Build history of the part. All positions in model axes, mm. A direction names the side the tool comes from. Round coordinates to 2 decimals unless told otherwise and drop trailing zeros. Order: outer loops, then holes, each group sorted by start corner. A loop starts at its lowest first (then second) coordinate and runs counter-clockwise, first axis right, second up. Notation, with made-up numbers: (59, 46.5) -> (89, 46.5) arc R24 ccw to (89, 76.5) -> close; hole circle Ø8 at (58.5, 77.5). An arc over 180 degrees is marked (long way). Answer as a JSON object with one key per item and string values.
from build123d import *

# Parameters (mm, degrees)
SKETCH_W        = 60
SKETCH_H        = 30
PAD_DEPTH       = 18
SKETCH001_W     = 16
SKETCH001_H     = 22
POCKET_DEPTH    = 15
SKETCH002_W     = 16
SKETCH002_H     = 10
POCKET001_DEPTH = 5
SKETCH003_R     = 2.3
POCKET002_DEPTH = 10
FILLET_R        = 5
CHAMFER_SIZE    = 4
CHAMFER001_SIZE = 0.6
CHAMFER002_SIZE = 1
SKETCH004_R     = 4
POCKET003_DEPTH = 5
CHAMFER003_SIZE = 0.4
FILLET001_R     = 1


with BuildPart() as part:
    # Sketch (on XZ_Plane of Origin) → Pad (new body)
    with BuildSketch(Plane.XZ):
        Rectangle(SKETCH_W, SKETCH_H)
    extrude(amount=PAD_DEPTH)

    # Sketch001 (on Face6 of Pad) → Pocket (cut)
    with BuildSketch(Plane.XZ.offset(18)):
        with Locations((-10, -1)):
            Rectangle(SKETCH001_W, SKETCH001_H)
        with Locations((10, -1)):
            Rectangle(SKETCH001_W, SKETCH001_H)
    extrude(amount=-POCKET_DEPTH, mode=Mode.SUBTRACT)

    # Sketch002 (on Face13 of Pocket) → Pocket001 (cut)
    with BuildSketch(Plane.XY.offset(-12)):
        with Locations((-10, -13)):
            Rectangle(SKETCH002_W, SKETCH002_H)
        with Locations((10, -13)):
            Rectangle(SKETCH002_W, SKETCH002_H)
    extrude(amount=-POCKET001_DEPTH, mode=Mode.SUBTRACT)

    # Sketch003 (on Face4 of Pocket001) → Pocket002 (cut)
    with BuildSketch(Plane.XZ.offset(18)):
        with Locations((-24, 0)):
            Circle(SKETCH003_R)
        with Locations((24, 0)):
            Circle(SKETCH003_R)
    extrude(amount=-POCKET002_DEPTH, mode=Mode.SUBTRACT)

    # Fillet
    fillet_edges = [part.edges().sort_by_distance(p)[0] for p in [
        (30, -9, -15),
        (30, -9, 15),
        (-30, -9, 15),
        (-30, -9, -15),
    ]]
    fillet(fillet_edges, radius=FILLET_R)

    # Chamfer
    chamfer_edges = [part.edges().sort_by_distance(p)[0] for p in [
        (0, -18, -15),
    ]]
    chamfer(chamfer_edges, length=CHAMFER_SIZE)

    # Chamfer001
    chamfer001_edges = [part.edges().sort_by_distance(p)[0] for p in [
        (-26.3, -18, 0),
        (21.7, -18, 0),
    ]]
    chamfer(chamfer001_edges, length=CHAMFER001_SIZE)

    # Chamfer002
    chamfer002_edges = [part.edges().sort_by_distance(p)[0] for p in [
        (-21.5, -18, -15),
    ]]
    chamfer(chamfer002_edges, length=CHAMFER002_SIZE)

    # Sketch004 → Pocket003 (cut)
    with BuildSketch(Plane.XZ.offset(3)):
        with Locations((-10, 0)):
            Circle(SKETCH004_R)
        with Locations((10, 0)):
            Circle(SKETCH004_R)
    extrude(amount=-POCKET003_DEPTH, mode=Mode.SUBTRACT)

    # Chamfer003
    chamfer003_edges = [part.edges().sort_by_distance(p)[0] for p in [
        (0, 0, -15),
        (-28.535534, 0, -13.535534),
        (28.535534, 0, -13.535534),
        (-30, 0, 0),
        (30, 0, 0),
        (-28.535534, 0, 13.535534),
        (28.535534, 0, 13.535534),
        (0, 0, 15),
        (-14, 0, 0),
        (6, 0, 0),
    ]]
    chamfer(chamfer003_edges, length=CHAMFER003_SIZE)

    # Fillet001
    fillet001_edges = [part.edges().sort_by_distance(p)[0] for p in [
        (-2, -10.5, 10),
        (2, -10.5, 10),
        (18, -10.5, 10),
        (-18, -10.5, 10),
    ]]
    fillet(fillet001_edges, radius=FILLET001_R)


solid = part.part
1) Cut at D-D, the plane x = -24. Give the cut face in (y, z).
Checked values:
{"outline": "(-18, -14) -> (-17, -15) -> (-0.4, -15) -> (0, -14.6) -> (0, 14.6) -> (-0.4, 15) -> (-17, 15) -> (-18, 14) -> (-18, 2.9) -> (-17.4, 2.3) -> (-8, 2.3) -> (-8, -2.3) -> (-17.4, -2.3) -> (-18, -2.9) -> close"}
2) Cut at C-C, the plane y = -15. Give the cut face in (x, z).
Checked values:
{"outline": "(-30, -10) arc R5 ccw to (-25, -15) -> (-18, -15) -> (-18, 9) arc R1 cw to (-17, 10) -> (-3, 10) arc R1 cw to (-2, 9) -> (-2, -14) -> (2, -14) -> (2, 9) arc R1 cw to (3, 10) -> (17, 10) arc R1 cw to (18, 9) -> (18, -15) -> (25, -15) arc R5 ccw to (30, -10) -> (30, 10) arc R5 ccw to (25, 15) -> (-25, 15) arc R5 ccw to (-30, 10) -> close; hole circle Ø4.6 at (-24, 0); hole circle Ø4.6 at (24, 0)"}
3) Cut at A-A, the plane y = -4.5. Give the cut face in (x, z), plus the area to 3 significant figures.
Checked values:
{"outline": "(-30, -10) arc R5 ccw to (-25, -15) -> (25, -15) arc R5 ccw to (30, -10) -> (30, 10) arc R5 ccw to (25, 15) -> (-25, 15) arc R5 ccw to (-30, 10) -> close; hole (-18, -12) -> (-2, -12) -> (-2, 9) arc R1 ccw to (-3, 10) -> (-17, 10) arc R1 ccw to (-18, 9) -> close; hole (2, -12) -> (18, -12) -> (18, 9) arc R1 ccw to (17, 10) -> (3, 10) arc R1 ccw to (2, 9) -> close", "area": "1,080 mm²"}
4) Pull direction Z, two halves, no side cores. Call faces 1 (the face through (-27.996, -17.715, 13.063)), 2 (the face through (0, 0, 0)), 3 (the face through (6, -2, 0)): pulls with the +Z half, pulls with the -Z half, needs draft (parallel to the pull), parting line crosses it, or undercut.
Checked values:
{"face 1": "pulls with the +Z half", "face 2": "needs draft", "face 3": "undercut"}
5) Probe L1, parallel to X at y = -8.25, z = -5.75; L2, parallel to Z at x = 24, y = -14; L3, parallel to Z at x = -10, y = -1.6. List the from-to ranges inside material, lowest first. Write a range as from..to.
Checked values:
{"L1": "x = -30..-18, -2..2, 18..30", "L2": "z = -15..-2.3, 2.3..15", "L3": "z = -15..-4, 4..15"}
6) Flat gauge pins, fed straight in: pin 1 Ø2.5 at (x, z) = (23, -0.5) entering from -Y; pin 2 Ø2 at (x, y) = (10.5, -14.5) entering from -Z; pin 3 Ø3.5 at (x, z) = (-12.5, -14) entering from -Y; pin 4 Ø5 at (x, z) = (-10, 0) entering from -Y (1 decimal). Where does each tip first touch, or does it go through?
Checked values:
{"pin 1": "stops at y = -17.47", "pin 2": "stops at z = 10", "pin 3": "stops at y = -8", "pin 4": "passes through"}
7) Cut at B-B, the plane x = 10. Give the cut face in (y, z), plus the area to 3 significant figures.
Checked values:
{"outline": "(-18, 10) -> (-3, 10) -> (-3, 4) -> (-0.4, 4) -> (0, 4.4) -> (0, 14.6) -> (-0.4, 15) -> (-17, 15) -> (-18, 14) -> close; (-8, -15) -> (-0.4, -15) -> (0, -14.6) -> (0, -4.4) -> (-0.4, -4) -> (-3, -4) -> (-3, -12) -> (-8, -12) -> close", "area": "155 mm²"}
8) Which spindle directions (+Z, -Z, +X, -X, +Y, -Y) get a long thin tool onto all of the face, cutting with end or side? Do faces 4 (the face through (28, -9, 14)), 5 (the face through (-21.806, -12.766, 0.691)), 6 (the face through (0, -16, -13)). Say none if no direction does.
Checked values:
{"face 4": "+Z, +X, +Y, -Y", "face 5": "-Y", "face 6": "-Z, -Y"}
